Build history of the part. All positions in model axes, mm. Give positions to 0.01 mm unless a question says otherwise; leave off trailing zeros. Loops run counter-clockwise (first coordinate to the right, second up) from the corner with the lowest first, then second, coordinate; pieces in that order, holes last. Notation, with made-up numbers: (15, 56) -> (35, 56) arc R13 ccw to (35, 61) -> close; hole circle Ø5 at (-34.75, 49.25). An arc over 180 degrees is marked (long way). Answer as a JSON object with one key per item and string values. Group by question number.
Q1. Band-saw the part on A-A, the plane x = 235. Write the cut outline in (y, z).
Q2. Drop flat-ended pins along their axis: pin 1 (1.5 mm diameter, centred on x = -119.5, y = -8, fed in from -Z); pin 2 (1.5 mm diameter, centred on x = -94, y = -8.5, fed in from -Z); pin 3 (4 mm diameter, centred on x = -4, y = -6.5, fed in from +Z). Give the stop position or say it passes through.
Q3. Wall check: probe 1 along Z at (x, y) = (135.5, -5.75); probe 2 along Z at (x, y) = (-30, -12); probe 3 along X at (y, z) = (-13.75, -151). Give the ranges that are in metal, low to high. Write a range as from..to.
from build123d import *

# Parameters (mm, degrees)
F1_DEPTH    = 18
F2_T1_DEPTH = 18


# Not quite as in the source:
# - a fillet or chamfer that OpenCascade refuses, or shapes differently, is made with other operations: its cross-section is extruded or revolved along the edge and cut away or added


with BuildPart() as f1:
    # F0 (on Front) → F1 (new body)
    with BuildSketch(Plane.XZ):
        with BuildLine():
            Line((295, -217), (-326, -217))
            add(Edge.make_bspline(
                [(85, -454), (9.4357049053, -467.1385897042), (-72.818934134, -466.1104352643), (-260.3771381726, -409.0142413584), (-323.4175443649, -304.8886355162), (-326, -217)],
                knots=[0, 0, 0, 0, 0.3230188863, 0.6489287258, 1, 1, 1, 1], degree=3))
            Line((85, -454), (85, -329))
            Line((85, -329), (295, -329))
            Line((295, -329), (295, -217))
        make_face()
        with BuildLine():
            add(Edge.make_bspline(
                [(85, 20), (9.4357049053, 33.1385897042), (-72.818934134, 32.1104352643), (-260.3771381726, -24.9857586416), (-323.4175443649, -129.1113644838), (-326, -217)],
                knots=[0, 0, 0, 0, 0.3230188863, 0.6489287258, 1, 1, 1, 1], degree=3))
            Line((-326, -217), (295, -217))
            Line((295, -217), (295, -105))
            Line((295, -105), (85, -105))
            Line((85, -105), (85, 20))
        make_face()
    extrude(amount=F1_DEPTH)

    # F2: fillet of radius 100 on 1 edges, made by hand

    # F2_s2 → F2_t1 (cut)
    with BuildSketch(Plane.XZ):
        with BuildLine():
            ThreePointArc((-325.8594220148, -221.0337656795), (-325.9408114638, -217), (-325.8594220148, -212.9662343205))
            Line((-325.8594220148, -212.9662343205), (-327.8577942258, -212.8855590069))
            ThreePointArc((-327.8577942258, -212.8855590069), (-327.9340315871, -214.9132915531), (-327.999137182, -216.9412588095))
            Line((-327.999137182, -216.9412588095), (-327.999137182, -217.0587411905))
            ThreePointArc((-327.999137182, -217.0587411905), (-327.9340315871, -219.0867084469), (-327.8577942258, -221.1144409931))
            Line((-327.8577942258, -221.1144409931), (-325.8594220148, -221.0337656795))
        make_face()
    extrude(amount=F2_T1_DEPTH, mode=Mode.SUBTRACT)


solid = f1.part
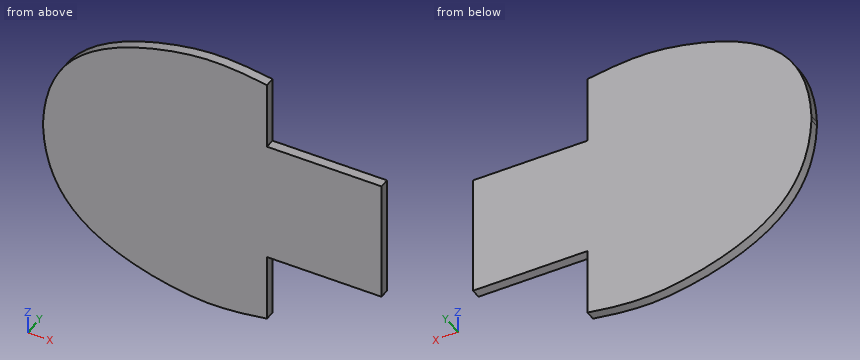
Worked answers:
{
 "1": {"outline": "(-18, -329) -> (0, -329) -> (0, -105) -> (-18, -105) -> close"},
 "2": {"pin 1": "z = -449.12", "pin 2": "z = -455.03", "pin 3": "z = 30.03"},
 "3": {"probe 1": "-329..-105", "probe 2": "-463.65..29.65", "probe 3": "-317.09..295"}
}
